Verification items for this drawing (mm, ordinates from the low corner). A direction names the side the tool comes from. Round coordinates to 2 decimals unless told otherwise and drop trailing zeros. Loops run counter-clockwise (first coordinate to the right, second up) from the corner with the lowest first, then second, coordinate; pieces in that order, holes last. Notation, with made-up numbers: (31, 10) -> (65, 10) arc R19 ccw to (65, 34) -> close; hole circle Ø1 at (-25.75, 79.5). An arc over 180 degrees is marked (long way). One line per item, written item: value. Start each with the question number.
1. Cross-section at B-B on z = 4.75. Record the cut outline in (x, y).
2. Cross-section at D-D on z = 6.5. Record the cut outline in (x, y).
3. Release check for a two-part mould opening along X. For the marked faces 3, 4 and 5 record: +X half, -X half, draft (parallel to the pull), parting line (faces both ways), or undercut.
4. Set-up check for the marked faces 1 and 2: record each of +Z, -Z, +X, -X, +Y, -Y from which the full face is reachable in a straight line by a thin tool's end or side.
5. Go/stop test with flat-tipped pins: pin 1 (2 mm diameter, centred on x = 13, y = 3, fed in from -Z); pin 2 (5 mm diameter, centred on y = 4, z = 11, fed in from -X); pin 3 (4 mm diameter, centred on x = 1.5, z = 8.5, fed in from +Y). Record where each tip stops, or that it passes through.
6. Material ranges on L1, parallel to X at y = 3.5, z = 6.5 (1 decimal); L2, parallel to Z at x = 2.25, y = 8.5 (1 decimal); L3, parallel to Z at x = 4.25, y = 8 (1 decimal), recorded low to high.
7. Cross-section at C-C on y = 8.5. Record the cut outline in (x, z) (1 decimal).
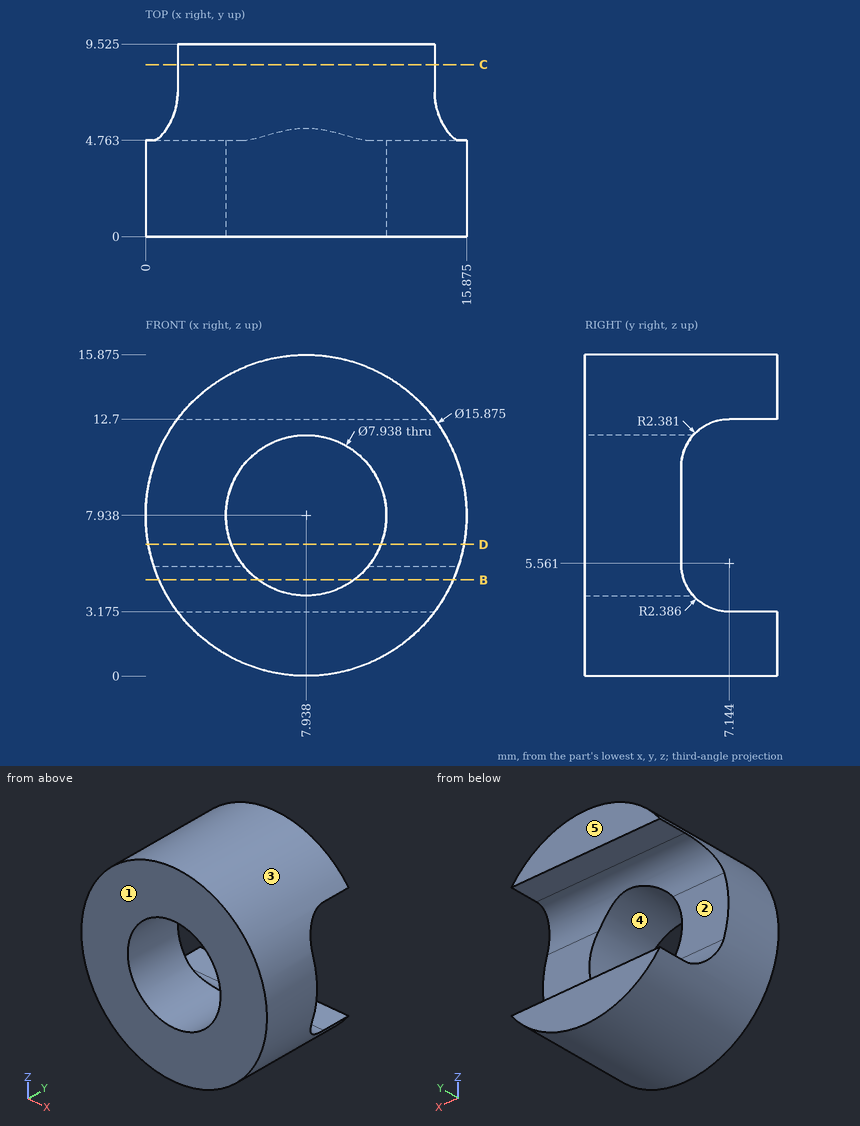
Taken from the geometry:
1. outline: (0.67, 0) -> (5.57, 0) -> (5.57, 4.9) -> (0.67, 4.9) -> close; (10.3, 0) -> (15.21, 0) -> (15.21, 4.9) -> (10.3, 4.9) -> close
2. outline: (0.13, 0) -> (4.24, 0) -> (4.24, 4.76) -> (0.13, 4.76) -> close; (11.64, 0) -> (15.74, 0) -> (15.74, 4.76) -> (11.64, 4.76) -> close
3. face 3: parting line
3. face 4: undercut
3. face 5: draft
4. face 1: +Z, -Z, +X, -X, -Y
4. face 2: +X, -X, +Y
5. pin 1: stops at z = 1.12
5. pin 2: stops at x = 0.02
5. pin 3: stops at y = 4.77
6. L1: x = 0.1 to 4.2, 11.6 to 15.7
6. L2: z = 2.4 to 3.2, 12.7 to 13.5
6. L3: z = 0.9 to 3.2, 12.7 to 15
7. outline: (1.6, 3.2) arc R7.9 ccw to (14.3, 3.2) -> close; (1.6, 12.7) -> (14.3, 12.7) arc R7.9 ccw to start
